from build123d import *
from build123d.topology import SkipClean

# Parameters (mm, degrees)
ESQUISSE1_R             = 2.5
BOSS_EXTRU_1_DEPTH      = 32
CHANFREIN1_SIZE         = 2
CONG_2_R                = 1
ENL_V_MAT_EXTRU_1_DEPTH = 2
ENL_V_START             = -20
ENL_V_MAT_EXTRU_2_DEPTH = 20
ENL_V_MAT_EXTRU_3_DEPTH = 53.991744678


with BuildPart() as part:
    # Esquisse1 → Boss.-Extru.1 (new body)
    with BuildSketch(Plane.XY):
        with BuildLine():
            Line((13.4187369, 3), (17.494642037, 3))
            ThreePointArc((17.494642037, 3), (11.441426921, 13.570418195), (0, 17.75))
            Line((0, 17.75), (-45.75, 17.75))
            Line((-45.75, 17.75), (-45.75, -17.75))
            Line((-45.75, -17.75), (0, -17.75))
            ThreePointArc((0, -17.75), (11.441426921, -13.570418195), (17.494642037, -3))
            Line((17.494642037, -3), (13.4187369, -3))
            ThreePointArc((13.4187369, -3), (-13.75, 0), (13.4187369, 3))
        make_face()
        with Locations((-37, 0)):
            Circle(ESQUISSE1_R, mode=Mode.SUBTRACT)
        with Locations((-27, 0)):
            Circle(ESQUISSE1_R, mode=Mode.SUBTRACT)
    extrude(amount=BOSS_EXTRU_1_DEPTH)

    # Chanfrein1
    chanfrein1_edges = [part.edges().sort_by_distance(p)[0] for p in [
        (-13.75, 0, 0),
    ]]
    chamfer(chanfrein1_edges, length=CHANFREIN1_SIZE)

    # Congé2
    cong_2_edges = [part.edges().sort_by_distance(p)[0] for p in [
        (17.494642037, -3, 16),
        (17.494642037, 3, 16),
        (13.4187369, -3, 17),
        (13.4187369, 3, 17),
    ]]
    fillet(cong_2_edges, radius=CONG_2_R)

    # Esquisse2 → Enlèv. mat.-Extru.1 (cut)
    with BuildSketch(Plane(origin=(0, 0, 0), x_dir=(-1, 0, 0), z_dir=(0, 0, -1))):
        with BuildLine():
            Line((45.75, 10.1), (27, 10.1))
            ThreePointArc((27, 10.1), (16.9, 0), (27, -10.1))
            Line((27, -10.1), (45.75, -10.1))
            Line((45.75, -10.1), (45.75, 10.1))
        make_face()
    extrude(amount=-ENL_V_MAT_EXTRU_1_DEPTH, mode=Mode.SUBTRACT)

    # Esquisse3 → Enlèv. mat.-Extru.2 (cut)
    with SkipClean():  # the faces are left unmerged after this step: merging them gives an invalid solid
        with BuildSketch(Plane.XY.offset(32).offset(ENL_V_START)):
            with BuildLine():
                Line((0, 17.75), (-45.75, 17.75))
                Line((-45.75, 17.75), (-45.75, -17.75))
                Line((-45.75, -17.75), (0, -17.75))
                ThreePointArc((0, -17.75), (-17.75, 0), (0, 17.75))
            make_face()
        extrude(amount=ENL_V_MAT_EXTRU_2_DEPTH, mode=Mode.SUBTRACT)

    # Esquisse5 → Enlèv. mat.-Extru.3 (cut, through all)
    with SkipClean():  # the faces are left unmerged after this step: merging them gives an invalid solid
        with BuildSketch(Plane.XY.offset(12)):
            Polygon((-15.75, 17.75), (-45.75, 10.75), (-45.75, 17.75), align=None)
            Polygon((-45.75, -17.75), (-15.75, -17.75), (-45.75, -10.75), align=None)
        extrude(amount=-ENL_V_MAT_EXTRU_3_DEPTH, mode=Mode.SUBTRACT)


solid = part.part
Geometry check sheet. Reference: the model listing, model coordinates, mm. A direction names the side the tool comes from. Round coordinates to 2 decimals unless told otherwise and drop trailing zeros. Loops run counter-clockwise (first coordinate to the right, second up) from the corner with the lowest first, then second, coordinate; pieces in that order, holes last. Notation, with made-up numbers: (58.25, 18.5) -> (63.25, 18.5) arc R20 ccw to (63.25, 51.5) -> close; hole circle Ø7 at (-39.75, 39.5). An arc over 180 degrees is marked (long way). Answer as a JSON object with one key per item and string values. Group by question number.
Item 1: Cross-section at B-B, the plane y = 0. Record the cut outline in (x, z), plus the area to 3 significant figures.
Item 2: Cross-section at C-C, the plane x = -37. Record the cut outline in (y, z), plus the area to 3 significant figures.
Item 3: Cross-section at D-D, the plane z = 30.5. Record the cut outline in (x, y), plus the area to 3 significant figures.
Item 4: Cross-section at A-A, the plane z = 4. Record the cut outline in (x, y).
Item 5: Release check for a two-part mould opening along X. For faces 4 (the face through (-30.54, 14.3, 6.08)), 5 (the face through (-13.74, -0.55, 16.79)), 6 (the face through (-36, -10.1, 1)) record: pulls with the +X half, pulls with the -X half, needs draft (parallel to the pull), parting line crosses it, or undercut.
Item 6: Thickness scan on line 1 along X through (y, z) = (0, 8.25); line 2 along Z through (x, y) = (-20.5, 0.5); line 3 along X through (y, z) = (0, 24). Record the ranges inside material, lowest first.
Item 7: Depth check by flat-ended pin: pin 1 Ø1 at (x, z) = (15.5, 8.5) entering from -Y; pin 2 Ø6 at (y, z) = (-13, 10) entering from +X (3 decimals); pin 3 Ø8 at (x, z) = (-21, 7) entering from +Y. Enter the tip coordinate at first touch or a pass-through.
Item 8: Set-up check for faces 1 (the face through (-16.9, 0.2, 1)), 2 (the face through (15, 3, 16)), 3 (the face through (-30.54, -14.3, 6.08)): record each of +Z, -Z, +X, -X, +Y, -Y from which the full face is reachable in a straight line by a thin tool's end or side.
Determined:
{
 "1": {"outline": "(-45.75, 2) -> (-39.5, 2) -> (-39.5, 12) -> (-45.75, 12) -> close; (-34.5, 2) -> (-29.5, 2) -> (-29.5, 12) -> (-34.5, 12) -> close; (-24.5, 2) -> (-16.9, 2) -> (-16.9, 0) -> (-15.75, 0) -> (-13.75, 2) -> (-13.75, 32) -> (-17.75, 32) -> (-17.75, 12) -> (-24.5, 12) -> close", "area": "304 mm²"},
 "2": {"outline": "(-12.79, 0) -> (-10.1, 0) -> (-10.1, 2) -> (-2.5, 2) -> (-2.5, 12) -> (-12.79, 12) -> close; (2.5, 2) -> (10.1, 2) -> (10.1, 0) -> (12.79, 0) -> (12.79, 12) -> (2.5, 12) -> close", "area": "217 mm²"},
 "3": {"outline": "(13.23, -3.73) arc R13.75 cw (long way) to (13.23, 3.73) arc R1 ccw to (14.2, 3) -> (16.27, 3) arc R1 ccw to (17.24, 4.24) arc R17.75 ccw (long way) to (17.24, -4.24) arc R1 ccw to (16.27, -3) -> (14.2, -3) arc R1 ccw to start", "area": "371 mm²"},
 "4": {"outline": "(-45.75, -10.75) -> (-15.75, -17.75) -> (0, -17.75) arc R17.75 ccw to (17.24, -4.24) arc R1 ccw to (16.27, -3) -> (14.2, -3) arc R1 ccw to (13.23, -3.73) arc R13.75 cw (long way) to (13.23, 3.73) arc R1 ccw to (14.2, 3) -> (16.27, 3) arc R1 ccw to (17.24, 4.24) arc R17.75 ccw to (0, 17.75) -> (-15.75, 17.75) -> (-45.75, 10.75) -> close; hole circle Ø5 at (-37, 0); hole circle Ø5 at (-27, 0)"},
 "5": {"face 4": "pulls with the -X half", "face 5": "undercut", "face 6": "needs draft"},
 "6": {"line 1": "x = -45.75 to -39.5, -34.5 to -29.5, -24.5 to -13.75", "line 2": "z = 2 to 12", "line 3": "x = -17.75 to -13.75"},
 "7": {"pin 1": "stops at y = -9.49", "pin 2": "stops at x = 14.665", "pin 3": "stops at y = 17.46"},
 "8": {"face 1": "-Z, -X", "face 2": "+Z, -Z, +X", "face 3": "+Z, -Z, -X, -Y"}
}
